from build123d import *

# Parameters (mm, degrees)
SKETCH1_R           = 14
BOSS_EXTRUDE1_DEPTH = 18
SKETCH2_R           = 1.45
CUT_EXTRUDE1_DEPTH  = 15
SKETCH3_R           = 1.4
CUT_EXTRUDE2_DEPTH  = 6
CIRPATTERN1_COUNT   = 8
SKETCH5_R           = 2.25
CUT_EXTRUDE3_DEPTH  = 15
CIRPATTERN2_COUNT   = 8
SKETCH6_R           = 4
BOSS_EXTRUDE2_DEPTH = 19
SKETCH7_R           = 8.5
CUT_EXTRUDE4_DEPTH  = 10
SKETCH8_R           = 7.75
SKETCH8_R_2         = 4.75
CUT_EXTRUDE5_DEPTH  = 5
SKETCH10_R          = 3.25
CUT_EXTRUDE6_DEPTH  = 2.5


with BuildPart() as part:
    # Sketch1 → Boss-Extrude1 (new body)
    with BuildSketch(Plane.XY):
        Circle(SKETCH1_R)
    extrude(amount=BOSS_EXTRUDE1_DEPTH)

    # Sketch2 → Cut-Extrude1 (cut)
    with BuildSketch(Plane.XY.offset(18)):
        with Locations((4.655041669, 4.170502016)):
            Circle(SKETCH2_R)
    extrude(amount=-CUT_EXTRUDE1_DEPTH, mode=Mode.SUBTRACT)

    # Sketch3 → Cut-Extrude2 (cut)
    with BuildSketch(Plane.XY.offset(18)):
        with Locations((0, 11)):
            Circle(SKETCH3_R)
    cut_extrude2 = extrude(amount=-CUT_EXTRUDE2_DEPTH, mode=Mode.SUBTRACT)

    # CirPattern1: Cut-Extrude2 ×8 about axis
    cirpattern1_axis = Axis((0, 0, 0), (0, 0, 1))
    for i in range(1, CIRPATTERN1_COUNT):
        add(cut_extrude2.rotate(cirpattern1_axis, i * 360 / CIRPATTERN1_COUNT), mode=Mode.SUBTRACT)

    # Sketch5 → Cut-Extrude3 (cut)
    with BuildSketch(Plane(origin=(0, 0, 0), x_dir=(-1, 0, 0), z_dir=(0, 0, -1))):
        with Locations((0, 11)):
            Circle(SKETCH5_R)
    cut_extrude3 = extrude(amount=-CUT_EXTRUDE3_DEPTH, mode=Mode.SUBTRACT)

    # CirPattern2: Cut-Extrude3 ×8 about axis
    cirpattern2_axis = Axis((0, 0, 0), (0, 0, 1))
    for i in range(1, CIRPATTERN2_COUNT):
        add(cut_extrude3.rotate(cirpattern2_axis, i * 360 / CIRPATTERN2_COUNT), mode=Mode.SUBTRACT)

    # Sketch6 → Boss-Extrude2 (add)
    with BuildSketch(Plane(origin=(0, 0, 0), x_dir=(-1, 0, 0), z_dir=(0, 0, -1))):
        Circle(SKETCH6_R)
    extrude(amount=BOSS_EXTRUDE2_DEPTH)

    # Sketch7 → Cut-Extrude4 (cut)
    with BuildSketch(Plane.XY.offset(18)):
        Circle(SKETCH7_R)
    extrude(amount=-CUT_EXTRUDE4_DEPTH, mode=Mode.SUBTRACT)

    # Sketch8 → Cut-Extrude5 (cut)
    with BuildSketch(Plane(origin=(0, 0, 0), x_dir=(-1, 0, 0), z_dir=(0, 0, -1))):
        Circle(SKETCH8_R)
        Circle(SKETCH8_R_2, mode=Mode.SUBTRACT)
    extrude(amount=-CUT_EXTRUDE5_DEPTH, mode=Mode.SUBTRACT)

    # Sketch9 → Revolve1 (revolve)
    with BuildSketch(Plane(origin=(0, 0, 0), x_dir=(1, 0, 0), z_dir=(0, 1, 0))):
        Polygon((4, 1.55754099), (4.75, 0), (4, 0), align=None)
    revolve(axis=Axis((0, 0, 18), (0, 0, -1)))

    # Sketch10 → Cut-Extrude6 (cut)
    with BuildSketch(Plane(origin=(0, 0, -19), x_dir=(-1, 0, 0), z_dir=(0, 0, -1))):
        Circle(SKETCH10_R)
    extrude(amount=-CUT_EXTRUDE6_DEPTH, mode=Mode.SUBTRACT)


solid = part.part
For this review, take the finished solid that the model builds, in its own axes (mm). A direction names the side the tool comes from. Give positions to 0.01 mm unless a question says otherwise; leave off trailing zeros. Order: outer loops, then holes, each group sorted by start corner. A loop starts at its lowest first (then second) coordinate and runs counter-clockwise, first axis right, second up. Notation, with made-up numbers: M 84.5,65 L 125.5,65 A29 ccw 125.5,103 Z; hole C -11,16 d8. An arc over 180 degrees is marked long. Answer in a Markdown table with one row per item. Add a question column.
(1) For faces 1 (the face through (1.009, 7.684, 2.465)), 2 (the face through (6.597, 7.026, 16.521)), 3 (the face through (4.57, 7.167, 13.07)), list the 3-axis set-ups (+Z, -Z, +X, -X, +Y, -Y) from which the entire face can be reached by the end or side of a thin tool; tool diameter is ignored.
(2) Consider section A-A on x = -11. State the section outline as (y, z) points, and give its area (3 significant figures).
(3) For pin 1 (5 mm diameter, centred on x = -2.5, y = 8, fed in from -Z); pin 2 (10 mm diameter, centred on x = 8.5, z = 2, fed in from +Y); pin 3 (10 mm diameter, centred on y = -7.5, z = 10, fed in from +X) (3 decimals), all flat-tipped, find the tip position at first contact; note any pin that passes through.
(4) Wall thickness on probe 1 along Y at (x, z) = (-6, 14.5); probe 2 along Y at (x, z) = (6.25, 3); probe 3 along Z at (x, y) = (-5.5, -1): over which ranges is each line inside the solid? List them lowest first. Write a range as [from, to].
(5) Consider section B-B on z = 13.5. Give the number of separate pieces and of enclosed holes in the cut face, and give its area (3 significant figures).
(6) Mouldability with a two-part tool opening along X and no side actions: class faces 4 (the face through (0.29, 13.23, 7.4)), 5 (the face through (0.867, -3.905, -10.157)) as +X half, -X half, draft (parallel to the pull), parting line (faces both ways), or undercut.
Evaluation:
| question | item | result |
|---|---|---|
| 1 | face 1 | -Z |
| 1 | face 2 | +Z, -Z |
| 1 | face 3 | +Z |
| 2 | outline | M -8.66,0 L -2.25,0 L -2.25,15 L -1.4,15 L -1.4,18 L -8.66,18 Z; M 1.4,15 L 2.25,15 L 2.25,0 L 8.66,0 L 8.66,18 L 1.4,18 Z |
| 2 | area | 236 mm^2 |
| 3 | pin 1 | stops at z = 0 |
| 3 | pin 2 | stops at y = 13.56 |
| 3 | pin 3 | stops at x = 13.775 |
| 4 | probe 1 | y = [-12.65, -9.16], [-6.4, -6.02], [6.02, 6.4], [9.16, 12.65] |
| 4 | probe 2 | y = [-12.53, -9.43], [-6.13, -4.58], [4.58, 6.13], [9.43, 12.53] |
| 4 | probe 3 | z = [5, 8] |
| 5 | separate pieces | 1 |
| 5 | enclosed holes | 9 |
| 5 | area | 262 mm^2 |
| 6 | face 4 | undercut |
| 6 | face 5 | parting line |
